from build123d import *

# Parameters (mm, degrees)
EXTRUDE1_DEPTH = 0.6
FILLET1_R      = 0.72


with BuildPart() as part:
    # Sketch1 → Extrude1 (new body, symmetric)
    with BuildSketch(Plane(origin=(0, 0, 0), x_dir=(0, 0, -1), z_dir=(1, 0, 0))):
        with BuildLine():
            Line((-8.710253959, -4.599345167), (-2.751581364, -3.12))
            ThreePointArc((-2.751581364, -3.12), (-1.470782105, -3.891323682), (0, -4.16))
            Line((0, -4.16), (0, -7.230967742))
            ThreePointArc((0, -7.230967742), (4.111002655, -5.948659652), (6.763950966, -2.556533162))
            Line((6.763950966, -2.556533162), (3.891323682, -1.470782105))
            ThreePointArc((3.891323682, -1.470782105), (4.16, 0), (3.891323682, 1.470782105))
            Line((3.891323682, 1.470782105), (6.763950966, 2.556533162))
            ThreePointArc((6.763950966, 2.556533162), (4.111002655, 5.948659652), (0, 7.230967742))
            Line((0, 7.230967742), (0, 4.16))
            ThreePointArc((0, 4.16), (-1.470782105, 3.891323682), (-2.751581364, 3.12))
            Line((-2.751581364, 3.12), (-8.710253959, 4.599345167))
            ThreePointArc((-8.710253959, 4.599345167), (9.85, 0), (-8.710253959, -4.599345167))
        make_face()
    extrude(amount=EXTRUDE1_DEPTH, both=True)

    # Fillet1
    fillet1_edges = [part.edges().sort_by_distance(p)[0] for p in [
        (0, -4.599345167, 8.710253959),
        (0, -7.230967742, 0),
        (0, -2.556533162, -6.763950966),
        (0, 2.556533162, -6.763950966),
        (0, 7.230967742, 0),
        (0, 4.599345167, 8.710253959),
    ]]
    fillet(fillet1_edges, radius=FILLET1_R)


solid = part.part
Input: part model. Units: mm. Frame: model coordinates. A direction names the side the tool comes from. Give positions to 0.01 mm unless a question says otherwise; leave off trailing zeros. Loops run counter-clockwise (first coordinate to the right, second up) from the corner with the lowest first, then second, coordinate; pieces in that order, holes last. Notation, with made-up numbers: (49, -21) -> (100, -21) arc R14 ccw to (100, 3) -> close; hole circle Ø5 at (21.5, -3). An arc over 180 degrees is marked (long way). Answer as a JSON object with one key per item and string values. Group by question number.
Item 1: Cut plane A-A, the plane x = -0.1. Return the cut outline in (y, z).
Item 2: Cut plane B-B, the plane z = 2.25. Return the cut outline in (x, y).
Item 3: Line query: probe 1 along Y at (x, z) = (0.25, -5.5); probe 2 along Y at (x, z) = (0.2, 5.5); probe 3 along Z at (x, y) = (0.2, -6.25). Output: solid intervals per line, ascending.
Item 4: Cut plane D-D, the plane z = 5. Return the cut outline in (x, y), and give its area (3 significant figures).
Item 5: Cut plane C-C, the plane y = -7.5. Return the cut outline in (x, z), and give its area (3 significant figures).
Item 6: Reachability of faces 1 (the flat face through (0.008, -3.752, 5.296)), 2 (the flat face through (0.6, 0, -5)), 3 (the flat face through (0, -5, 0)) from +Z, -Z, +X, -X, +Y, -Y: full face, straight path, thin tool, end or side. Return the list, or none.
Item 7: Pull-direction query (Y, two-part tool) for faces 4 (the cylindrical face through (0.01, 3.9, 1.45)), 5 (the flat face through (-0.6, 0, -5)), 6 (the cylindrical face through (0.01, 5.92, -4.15)), 7 (the cylindrical face through (0.008, 0.352, -9.844)); classes: released by +Y, released by -Y, zero draft, split by the parting line, or undercut.
Checks:
{
 "1": {"outline": "(-7.19, -0.8) arc R0.72 cw to (-6.47, 0) -> (-4.16, 0) arc R4.16 cw to (-3.12, 2.75) -> (-4.37, 7.77) arc R0.72 ccw to (-5.46, 8.2) arc R9.85 ccw (long way) to (5.46, 8.2) arc R0.72 ccw to (4.37, 7.77) -> (3.12, 2.75) arc R4.16 cw to (4.16, 0) -> (6.47, 0) arc R0.72 cw to (7.19, -0.8) arc R7.23 cw to (3.29, -6.44) arc R0.72 cw to (2.29, -6.05) -> (1.47, -3.89) arc R4.16 cw to (-1.47, -3.89) -> (-2.29, -6.05) arc R0.72 cw to (-3.29, -6.44) arc R7.23 cw to start"},
 "2": {"outline": "(-0.6, -9.59) -> (0.6, -9.59) -> (0.6, -3.5) -> (-0.6, -3.5) -> close; (-0.6, 3.5) -> (0.6, 3.5) -> (0.6, 9.59) -> (-0.6, 9.59) -> close"},
 "3": {"probe 1": "y = -8.17 to -4.69, -2.08 to 2.08, 4.69 to 8.17", "probe 2": "y = -8.17 to -3.8, 3.8 to 8.17", "probe 3": "z = -7.61 to -3.64, 0 to 7.61"},
 "4": {"outline": "(-0.6, -8.49) -> (0.6, -8.49) -> (0.6, -3.68) -> (-0.6, -3.68) -> close; (-0.6, 3.68) -> (0.6, 3.68) -> (0.6, 8.49) -> (-0.6, 8.49) -> close", "area": "11.5 mm²"},
 "5": {"outline": "(-0.6, -6.39) -> (0.6, -6.39) -> (0.6, 6.39) -> (-0.6, 6.39) -> close", "area": "15.3 mm²"},
 "6": {"face 1": "+Z, +X, -X", "face 2": "+Z, -Z, +X, +Y, -Y", "face 3": "+X, -X"},
 "7": {"face 4": "undercut", "face 5": "zero draft", "face 6": "undercut", "face 7": "split by the parting line"}
}
